Autodesk Fusion 360 part; units mm, degrees
sketch "Sketch1" plane through (0, 0, 0) normal (0, 0, 1) x (1, 0, 0)
  line L0 (-27.6756, 45.9596) -> (34.3244, 45.9596)
  line L1 (-32.6756, 40.9596) -> (-32.6756, -84.0404)
  line L2 (-27.6756, -89.0404) -> (34.3244, -89.0404)
  line L3 (39.3244, -84.0404) -> (39.3244, 40.9596)
  arc A0 (39.3244, 40.9596) -> (34.3244, 45.9596) centre (34.3244, 40.9596) ccw
  arc A1 (-27.6756, 45.9596) -> (-32.6756, 40.9596) centre (-27.6756, 40.9596) ccw
  arc A2 (-32.6756, -84.0404) -> (-27.6756, -89.0404) centre (-27.6756, -84.0404) ccw
  arc A3 (34.3244, -89.0404) -> (39.3244, -84.0404) centre (34.3244, -84.0404) ccw
  circle A4 centre (-27.6756, 40.9596) radius 1.6
  circle A5 centre (34.3244, 40.9596) radius 1.6
  circle A6 centre (34.3244, -84.0404) radius 1.6
  circle A7 centre (-27.6756, -84.0404) radius 1.6
  circle A8 centre (3.3244, 35.9596) radius 2.5
  circle A9 centre (-16.6756, 41.9596) radius 1.6
  circle A10 centre (-16.6756, 29.9596) radius 1.6
  circle A11 centre (23.3244, 41.9596) radius 1.6
  circle A12 centre (23.3244, 29.9596) radius 1.6
  line L4 (-9.1756, 20.9596) -> (-9.1756, -35.0404)
  line L5 (-9.1756, 20.9596) -> (15.8244, 20.9596)
  line L6 (15.8244, 20.9596) -> (15.8244, -35.0404)
  line L7 (-9.1756, -35.0404) -> (15.8244, -35.0404)
  line L8 (-17.4618, -35.0396) -> (-17.4618, -71.7396)
  line L9 (-17.4618, -71.7396) -> (23.5382, -71.7396)
  line L10 (23.5382, -71.7396) -> (23.5382, -35.0396)
  line L11 (-17.4618, -35.0396) -> (23.5382, -35.0396)
  line L12 (-28.8687, -53.3412) -> (-21.2687, -53.3412)
  line L13 (-28.8687, -53.3412) -> (-28.8687, -60.9412)
  line L14 (-21.2687, -53.3412) -> (-21.2687, -60.9412)
  line L15 (-28.8687, -60.9412) -> (-21.2687, -60.9412)
  line L16 (-60, -39) -> (-60, -28)
  line L17 (-17.4618, -71.7396) -> (-17.4618, -60.7396)
  line L18 (-17.4618, -60.7396) -> (-0.4618, -60.7396)
  line L19 (-17.4618, -71.7396) -> (-0.4618, -71.7396)
  line L20 (-17.4618, -53.3896) -> (-0.4625, -53.5429)
  line L21 (-0.4625, -53.5429) -> (-0.3813, -44.5432)
  line L22 (-0.3813, -44.5432) -> (-17.4618, -44.5432)
  line L23 (-17.4618, -44.5432) -> (-17.4618, -53.3896)
  line L24 (18.5382, -71.7396) -> (18.5382, -67.7396)
  line L25 (18.5382, -67.7396) -> (0.5382, -67.7396)
  line L26 (0.5382, -71.7396) -> (18.5382, -71.7396)
  line L27 (0.5382, -67.7396) -> (-0.4618, -67.7396)
  line L28 (-0.4618, -60.7396) -> (-0.4618, -67.7396)
  line L29 (27.6313, -53.3412) -> (35.2313, -53.3412)
  line L30 (35.2313, -53.3412) -> (35.2313, -60.9412)
  line L31 (27.6313, -53.3412) -> (27.6313, -60.9412)
  line L32 (27.6313, -60.9412) -> (35.2313, -60.9412)
  point P0 (-32.6756, 45.9596)
  point P1 (39.3244, 45.9596)
  point P2 (-32.6756, -89.0404)
  point P3 (39.3244, -89.0404)
  point P4 (39.3244, 20.9596)
  dimension "d1" = 72
  dimension "d2" = 135
  dimension "d3" = 72
  dimension "d4" = 110
  dimension "d5" = 5
  dimension "d6" = 5
  dimension "d7" = 5
  dimension "d8" = 5
  dimension "d9" = 3.2
  dimension "d10" = 3.2
  dimension "d11" = 3.2
  dimension "d12" = 3.2
  dimension "d14" = 5
  dimension "d19" = 10
  dimension "d23" = 3.2
  dimension "d24" = 3.2
  dimension "d25" = 3.2
  dimension "d26" = 3.2
  dimension "d27" = 56
  dimension "d28" = 25
  dimension "d29" = 56
  dimension "d32" = 36.7
  dimension "d33" = 41
  dimension "d34" = 36.7
  dimension "d35" = 7.6
  dimension "d37" = 7.6
  dimension "d38" = 7.6
  dimension "d39" = 11
  dimension "d42" = 17
  dimension "d43" = 9
  dimension "d46" = 4
  dimension "d48" = 7.6
  dimension "d49" = 7.6
  dimension "d50" = 7.6
extrude "Extrude1" add sketch "Sketch1" along normal blind 3.5 contours L0 L1 L2 L3 A0 A1 A2 A3 | L8 L20 L21 L22 L23 | L8 L9 L17 L18 L19 L24 L25 L26 L27 L28 makes body 1
sketch "Sketch2" plane through (0, 0, 0) normal (1, 0, 0) x (0, 1, 0)
  circle A0 centre (-58.9237, 12.2782) radius 4
  circle A1 centre (-58.9237, 12.2782) radius 2.5
  dimension "d53" = 8
  dimension "d54" = 5
extrude "Extrude3" add sketch "Sketch2" along normal blind 72 separate body makes body 2
move_body "Align1" bodies 2 to x (0, -1, 0) y (1, 0, 0) z (0, 0, 1) at (26.2481, -58.9237, -8.7782)
move_body "Align2" bodies 2 to x (1, 0, 0) y (0, 1, 0) z (0, 0, 1) at (72, 0, 0)
move_body "Move3" bodies 2 to x (0, 1, 0) y (-1, 0, 0) z (0, 0, 1) at (-94.8493, -166.9981, 0)
move_body "Move4" bodies 2 to x (1, 0, 0) y (0, 1, 0) z (0, 0, 1) at (3.25, 70.5, 0)
move_body "Move5" bodies 2 to x (1, 0, 0) y (0, 1, 0) z (0, 0, 1) at (0, 0, -1.7)
combine "Combine1" operation add target body 1 tool bodies 2
sketch "Sketch3" plane through (0, 0, 0) normal (1, 0, 0) x (0, 1, 0)
  circle A0 centre (-60, 35) radius 2.5
  dimension "d59" = 5
extrude "Extrude4" add sketch "Sketch3" along normal blind 300 separate body makes body 3
move_body "Move6" bodies 3 to x (1, 0, 0) y (0, 1, 0) z (0, 0, 1) at (0, 2.5942, -33.2053)
move_body "Move7" bodies 3 to x (1, 0, 0) y (0, 1, 0) z (0, 0, 1) at (0, 0.23, 0)
move_body "Move8" bodies 3 to x (1, 0, 0) y (0, 1, 0) z (0, 0, 1) at (-60, 0, 0)
combine "Combine2" operation cut target body 1 tool bodies 3
extrude "Extrude5" add sketch "Sketch1" along normal blind 500 separate body contours L12 L13 L14 L15 makes body 4
move_body "Move9" bodies 4 to x (1, 0, 0) y (0, 1, 0) z (0, 0, 1) at (0, 0, -22)
combine "Combine3" operation cut target body 1 tool bodies 4
extrude "Extrude6" add sketch "Sketch1" along normal blind 500 separate body contours L29 L30 L31 L32 makes body 5
move_body "Move10" bodies 5 to x (1, 0, 0) y (0, 1, 0) z (0, 0, 1) at (0, 0, -14)
combine "Combine4" operation cut target body 1 tool bodies 5
extrude "Extrude7" cut sketch "Sketch1" along normal blind 30 contours L7 L8 L9 L10 L11 L18 L20 L21 L22 L24 L25 L27 L28 bodies 1
extrude "Extrude8" cut sketch "Sketch1" against normal blind 7 contours L7 L8 L9 L10 L11 L18 L20 L21 L22 L24 L25 L27 L28 bodies 1
sketch "Sketch6" plane through (0, 0, 0) normal (1, 0, 0) x (0, 1, 0)
  circle A0 centre (2.5, 8.5) radius 4
  circle A1 centre (2.5, 8.5) radius 2.5
  dimension "d70" = 8
  dimension "d71" = 5
extrude "Extrude9" add sketch "Sketch6" along normal blind 74 separate body makes body 6
sketch "Sketch7" plane through (0, 0, 3.5) normal (0, 0, 1) x (-1, 0, 0)
  line L0 (-23.5382, 53.5529) -> (-27.6313, 53.5529)
  line L1 (-27.6313, 53.5529) -> (-27.6313, 53.3412)
  line L2 (-27.6313, 53.3412) -> (-35.2313, 53.3412)
  line L3 (-35.2313, 53.3412) -> (-35.2313, 53.5529)
  line L4 (-35.2313, 53.5529) -> (-39.3244, 53.5529)
  line L5 (-39.3244, 53.5529) -> (-39.3244, -40.9596)
  arc A0 (-39.3244, -40.9596) -> (-34.3244, -45.9596) centre (-34.3244, -40.9596) ccw
  line L6 (-34.3244, -45.9596) -> (27.6756, -45.9596)
  arc A1 (27.6756, -45.9596) -> (32.6756, -40.9596) centre (27.6756, -40.9596) ccw
  line L7 (32.6756, -40.9596) -> (32.6756, 53.5529)
  line L8 (32.6756, 53.5529) -> (28.8687, 53.5529)
  line L9 (28.8687, 53.5529) -> (28.8687, 53.3412)
  line L10 (28.8687, 53.3412) -> (21.2687, 53.3412)
  line L11 (21.2687, 53.3412) -> (21.2687, 53.5529)
  line L12 (21.2687, 53.5529) -> (17.4618, 53.5529)
  line L13 (17.4618, 53.5529) -> (17.4618, 53.3896)
  line L14 (17.4618, 53.3896) -> (0.4625, 53.5429)
  line L15 (0.4625, 53.5429) -> (0.3813, 44.5432)
  line L16 (0.3813, 44.5432) -> (17.4618, 44.5432)
  line L17 (17.4618, 44.5432) -> (17.4618, 35.0396)
  line L18 (17.4618, 35.0396) -> (9.1756, 35.0396)
  line L19 (9.1756, 35.0396) -> (9.1756, -20.9596)
  line L20 (9.1756, -20.9596) -> (-15.8244, -20.9596)
  line L21 (-15.8244, -20.9596) -> (-15.8244, 35.0396)
  line L22 (-15.8244, 35.0396) -> (-23.5382, 35.0396)
  line L23 (-23.5382, 35.0396) -> (-23.5382, 53.5529)
  circle A2 centre (-23.3244, -29.9596) radius 1.6
  circle A3 centre (16.6756, -29.9596) radius 1.6
  circle A4 centre (-34.3244, -40.9596) radius 1.6
  circle A5 centre (16.6756, -41.9596) radius 1.6
  circle A6 centre (-3.3244, -35.9596) radius 2.5
  circle A7 centre (-23.3244, -41.9596) radius 1.6
  circle A8 centre (27.6756, -40.9596) radius 1.6
  line L24 (-15.8244, 35.0397) -> (-22.8244, 35.0397)
  line L25 (-22.8244, 35.0397) -> (-22.8244, -19.9603)
  line L26 (-22.8244, -19.9603) -> (-15.8244, -19.9603)
  line L27 (-15.8244, -19.9603) -> (-15.8244, 35.0397)
  dimension "d74" = 7
  dimension "d75" = 55
sketch "Sketch9" plane through (0, 0, 3.5) normal (0, 0, 1) x (1, 0, 0)
  line L0 (-9.1755, -35.0462) -> (-16.1755, -35.0462)
  line L1 (-16.1755, -35.0462) -> (-16.1755, 19.9538)
  line L2 (-16.1755, 19.9538) -> (-9.1755, 19.9538)
  line L3 (-9.1755, 19.9538) -> (-9.1755, -35.0462)
  dimension "d81" = 7
  dimension "d82" = 55
  dimension "d83" = 7
extrude "Extrude11" add sketch "Sketch9" sketch "Sketch7" along normal blind 9.75 of sketch 2 contours L21 L22 L24 L25 L26 L27 bodies 1
extrude "Extrude12" add sketch "Sketch9" sketch "Sketch7" against normal blind 13.25 of sketch 2 contours L21 L22 L24 L25 L26 L27 bodies 1
sketch "Sketch11" plane through (22.8244, 0, 0) normal (1, 0, 0) x (0, 1, 0)
  line L0 (-35.0396, 3.5) -> (19.9603, 3.5)
  line L1 (19.9603, 3.5) -> (19.9603, 13.25)
  line L2 (19.9603, 13.25) -> (-35.0396, 13.25)
  line L3 (-35.0396, 13.25) -> (-35.0396, 3.5)
  line L4 (-35.0396, 13.25) -> (-35.0284, 13.25) construction
  circle A0 centre (-30.5396, 8.75) radius 3.5
  line L5 (-35.0396, 8.75) -> (-30.5396, 8.75)
  line L6 (-30.5396, 8.75) -> (-30.5396, 13.25)
  line L7 (19.9603, 8.75) -> (15.4603, 8.75)
  line L8 (15.4603, 8.75) -> (15.4603, 13.25)
  circle A1 centre (15.4603, 8.75) radius 3.5
  dimension "d91" = 7
  dimension "d94" = 4.5
  dimension "d95" = 4.5
  dimension "d96" = 4.5
  dimension "d97" = 4.5
  dimension "d98" = 7
extrude "Extrude13" cut sketch "Sketch11" against normal blind 82 contours A0 L5 L6 | A0 L5 L6 | L7 L8 A1 | L7 L8 A1 bodies 1
sketch "Sketch12" plane through (22.8244, 0, 0) normal (1, 0, 0) x (0, 1, 0)
  line L0 (19.9603, 0) -> (-35.0396, 0)
  line L1 (-35.0396, 0) -> (-35.0396, -9.75)
  line L2 (-35.0396, -9.75) -> (19.9603, -9.75)
  line L3 (19.9603, -9.75) -> (19.9603, 0)
  line L4 (-35.0396, -5.25) -> (-30.5396, -5.25)
  line L5 (-30.5396, -5.25) -> (-30.5396, -9.75)
  circle A0 centre (-30.5396, -5.25) radius 3.5
  line L6 (15.5072, -9.75) -> (15.5072, -5.25)
  line L7 (15.5072, -5.25) -> (20.0072, -5.25)
  circle A1 centre (15.5072, -5.25) radius 3.5
  dimension "d101" = 4.5
  dimension "d102" = 4.5
  dimension "d103" = 7
  dimension "d104" = 4.5
  dimension "d105" = 4.5
  dimension "d106" = 7
extrude "Extrude14" cut sketch "Sketch12" against normal blind 1000 contours L6 L7 A1 | L6 L7 A1 | L4 L5 A0 | L4 L5 A0 bodies 1
extrude "Extrude10" [suppressed]
fillet "Fillet1" [suppressed]
hidden bodies 6
Read the model definition and answer for the solid it produces. Units are mm, in the model's axes. A direction names the side the tool comes from. Give positions to 0.01 mm unless a question says otherwise; leave off trailing zeros. Write each loop counter-clockwise with the first axis right and the second up, starting at its lowest first coordinate (ties: lowest second). Pieces come first, ordered by that corner, then holes. Notation, with made-up numbers: M 37,34 L 95,34 A19 ccw 95,56 Z; hole C 78,-17.5 d1. An arc over 180 degrees is marked long. Put each result on its own line as item: value. Start each with the question number.
1. The part is cut by section A-A, the plane y = -10. Give the vertices of the cut face in (x, z), and give its area (4 significant figures).
2. For a pull along X with two mould halves and no side action, classify faces 5 (the cylindrical face through (34.116, -85.627, 1.726)), 6 (the cylindrical face through (-12.6, -33.3, 6.6)), 7 (the flat face through (-32.676, -21, 1)) as released by +X, released by -X, zero draft, split by the parting line, or undercut.
3. Which of the six approach directions +Z, -Z, +X, -X, +Y, -Y give full straight-line access (tool end or side, diameter ignored) to faces 1 (the flat face through (35.231, -55, 0)), 2 (the flat face through (3, -75, 3.5)), 3 (the cylindrical face through (-30.8, -57.2, 4.3)), 4 (the flat face through (19, 19.96, -5))?
4. The part is cut by section D-D, the plane x = -6. Give the number of separate pieces and of enclosed holes in the cut face, and give its area (3 significant figures).
5. Each of these flat-tipped pins is pushed along its axis until it touches: pin 1 Ø2.5 at (x, z) = (18.5, 5.5) entering from -Y; pin 2 Ø9 at (y, z) = (15.46, 8.75) entering from +X; pin 3 Ø4 at (x, y) = (30.5, -33.5) entering from -Z. Where does it stop, or does it pass through?
6. The part is cut by section C-C, the plane z = -5.25. Give the vertices of the cut face in (x, y).
7. Consider line 1 along X through (y, z) = (-1.5, 8.25); line 2 along Y through (x, z) = (-14, 1.5); line 3 along X through (y, z) = (-9, 0.5). Determine where each line is inside the solid, lowest interval first.
8. The part is cut by section B-B, the plane x = 9. Give the vertices of the cut face in (y, z), and give its area (3 significant figures).
Final values:
1. outline: M -32.68,0 L -16.18,0 L -16.18,-9.75 L -9.18,-9.75 L -9.18,0 L -9.18,13.25 L -16.18,13.25 L -16.18,3.5 L -32.68,3.5 Z; M 15.82,-9.75 L 22.82,-9.75 L 22.82,0 L 39.32,0 L 39.32,3.5 L 22.82,3.5 L 22.82,13.25 L 15.82,13.25 Z
1. area: 437.5 mm²
2. face 5: undercut
2. face 6: zero draft
2. face 7: released by -X
3. face 1: +Z, -Z
3. face 2: +Z, +X, -X, -Y
3. face 3: +X, -X
3. face 4: -Z, +X, -X, +Y
4. separate pieces: 3
4. enclosed holes: 0
4. area: 218 mm²
5. pin 1: stops at y = -35.04
5. pin 2: stops at x = 22.82
5. pin 3: stops at z = 0
6. outline: M -16.18,-35.05 L -9.18,-35.05 L -9.18,-34.04 L -16.18,-34.04 Z; M -16.18,-27.04 L -9.18,-27.04 L -9.18,12.01 L -16.18,12.01 Z; M -16.18,19.01 L -9.18,19.01 L -9.18,19.95 L -16.18,19.95 Z; M 15.82,-35.04 L 22.82,-35.04 L 22.82,-34.04 L 15.82,-34.04 Z; M 15.82,-27.04 L 22.82,-27.04 L 22.82,12.01 L 15.82,12.01 Z; M 15.82,19.01 L 22.82,19.01 L 22.82,19.96 L 15.82,19.96 Z
7. line 1: x = -16.18 to -9.18, 15.82 to 22.82
7. line 2: y = -89.04 to -60.74, -53.42 to -44.54, -35.05 to 45.96
7. line 3: x = -32.68 to -9.18, 15.82 to 39.32
8. outline: M -89.04,0 L -67.74,0 L -67.74,3.5 L -89.04,3.5 Z; M 20.96,0 L 45.96,0 L 45.96,3.5 L 20.96,3.5 Z
8. area: 162 mm²
